```python
from build123d import *

# Parameters (mm, degrees)
ESBO_O1_W                = 195
ESBO_O1_H                = 115
RESSALTO_EXTRUS_O1_DEPTH = 10
ESBO_O2_W                = 32
ESBO_O2_H                = 7
ESBO_O2_W_2              = 7
ESBO_O2_H_2              = 32
CORTE_EXTRUS_O2_DEPTH    = 11
ESBO_O3_R                = 1.5
CORTE_EXTRUS_O3_DEPTH    = 11


with BuildPart() as part:
    # Esboço1 → Ressalto-extrusão1 (new body)
    with BuildSketch(Plane(origin=(0, 0, 0), x_dir=(1, 0, 0), z_dir=(0, 1, 0))):
        Rectangle(ESBO_O1_W, ESBO_O1_H)
    extrude(amount=RESSALTO_EXTRUS_O1_DEPTH)

    # Esboço2 → Corte-extrusão2 (cut, through all)
    with BuildSketch(Plane(origin=(0, 10, 0), x_dir=(1, 0, 0), z_dir=(0, 1, 0))):
        with Locations((-37.5, -52.5)):
            Rectangle(ESBO_O2_W, ESBO_O2_H)
        with Locations((37.5, -52.5)):
            Rectangle(ESBO_O2_W, ESBO_O2_H)
        with Locations((37.5, 52.5)):
            Rectangle(ESBO_O2_W, ESBO_O2_H)
        with Locations((-37.5, 52.5)):
            Rectangle(ESBO_O2_W, ESBO_O2_H)
        with Locations((-92.5, 23.75)):
            Rectangle(ESBO_O2_W_2, ESBO_O2_H_2)
        with Locations((-92.5, -23.75)):
            Rectangle(ESBO_O2_W_2, ESBO_O2_H_2)
        with Locations((92.5, -23.75)):
            Rectangle(ESBO_O2_W_2, ESBO_O2_H_2)
        with Locations((92.5, 23.75)):
            Rectangle(ESBO_O2_W_2, ESBO_O2_H_2)
    extrude(amount=-CORTE_EXTRUS_O2_DEPTH, mode=Mode.SUBTRACT)

    # Esboço3 → Corte-extrusão3 (cut, through all)
    with BuildSketch(Plane(origin=(0, 10, 0), x_dir=(1, 0, 0), z_dir=(0, 1, 0))):
        with Locations((-92.5, 52.5)):
            Circle(ESBO_O3_R)
        with Locations((92.5, 52.5)):
            Circle(ESBO_O3_R)
        with Locations((92.5, -52.5)):
            Circle(ESBO_O3_R)
        with Locations((-92.5, -52.5)):
            Circle(ESBO_O3_R)
    extrude(amount=-CORTE_EXTRUS_O3_DEPTH, mode=Mode.SUBTRACT)


solid = part.part
```
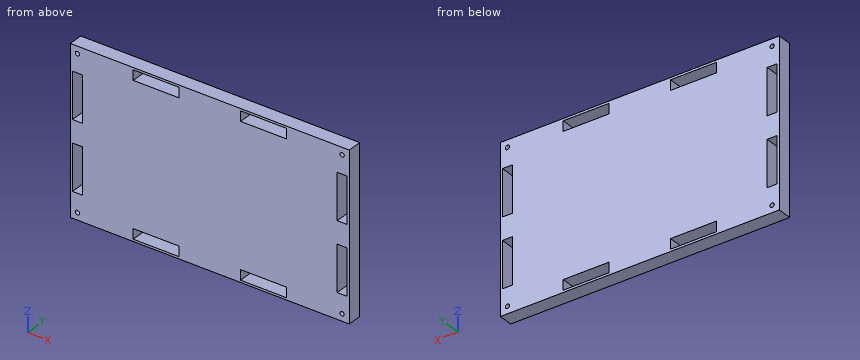
Here's how the part is built. I have some questions about the finished solid (model axes, mm). Give positions to 0.01 mm unless a question says otherwise; leave off trailing zeros. Write each loop counter-clockwise with the first axis right and the second up, starting at its lowest first coordinate (ties: lowest second). Pieces come first, ordered by that corner, then holes. Notation, with made-up numbers: M 78,36 L 85,36 A6 ccw 85,44 Z; hole C -32,74.5 d7. An arc over 180 degrees is marked long. Put each result on its own line as item: value. Start each with the question number.
Item 1: I need wall thicknesses on L1, parallel to Z at x = -92.5, y = 2.25; L2, parallel to X at y = 5.75, z = -52.5; L3, parallel to Z at x = 41, y = 8. Which ranges of each line are inside material? Lowest first, please. Write a range as from..to.
Item 2: If we section it at C-C, the plane y = 3.5: Count the separate pieces of the cut face and the enclosed holes in it, then the cut area to 3 significant figures.
Item 3: If we section it at A-A, the plane x = -37: Write out the boundary of the cut face in (y, z).
Item 4: If we section it at B-B, the plane z = -16: Write out the boundary of the cut face in (x, y), then the cut area to 3 significant figures.
Values:
1. L1: -57.5..-54, -51..-39.75, -7.75..7.75, 39.75..51, 54..57.5
1. L2: -97.5..-94, -91..-53.5, -21.5..21.5, 53.5..91, 94..97.5
1. L3: -57.5..-56, -49..49, 56..57.5
2. separate pieces: 1
2. enclosed holes: 12
2. area: 20,600 mm²
3. outline: M 0,-57.5 L 10,-57.5 L 10,-56 L 0,-56 Z; M 0,-49 L 10,-49 L 10,49 L 0,49 Z; M 0,56 L 10,56 L 10,57.5 L 0,57.5 Z
4. outline: M -97.5,0 L -96,0 L -96,10 L -97.5,10 Z; M -89,0 L 89,0 L 89,10 L -89,10 Z; M 96,0 L 97.5,0 L 97.5,10 L 96,10 Z
4. area: 1,810 mm²
